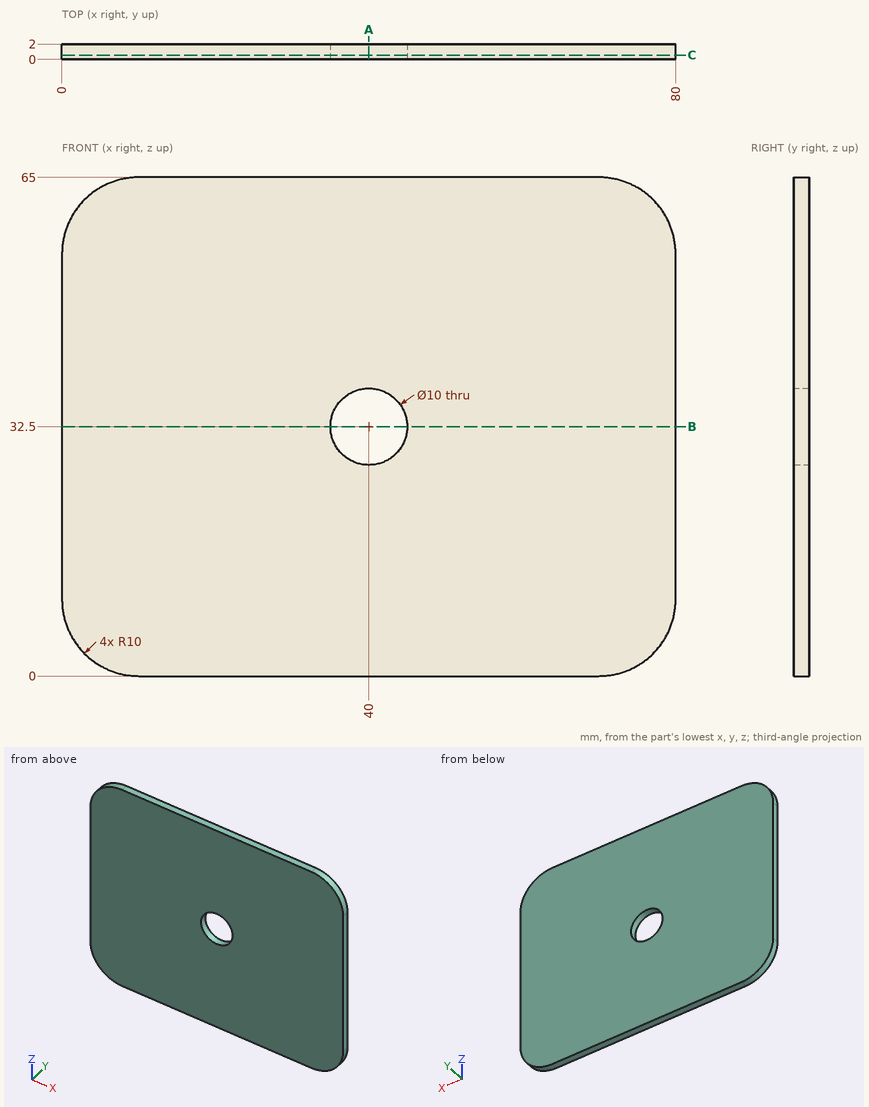
Design review of the part shown in the three views and the two pictorial views. Dimensions are in mm from the part's minimum x, y and z. Round coordinates to 2 decimals unless told otherwise and drop trailing zeros. Order: outer loops, then holes, each group sorted by start corner. A loop starts at its lowest first (then second) coordinate and runs counter-clockwise, first axis right, second up.
(1) For P1, Ø8, axis at x = 40, z = 32.5, coming from the -Y side, flat-tipped, find the tip position at first contact; note if it passes through.
Working result:
P1: passes through
(2) Take a section at A-A, the plane x = 40. State the section outline as (y, z) points, plus the area to 3 significant figures.
Working result:
outline: (0, 0) - (2, 0) - (2, 27.5) - (0, 27.5) - close; (0, 37.5) - (2, 37.5) - (2, 65) - (0, 65) - close
area: 110 mm2
(3) Wall thickness on L1, parallel to X at y = 1.3, z = 32.5; L2, parallel to Z at x = 37.5, y = 0.25; L3, parallel to Z at x = 6.5, y = 0.8: over which ranges is each line inside the solid? List them lowest first.
Working result:
L1: x = 0 to 35, 45 to 80
L2: z = 0 to 28.17, 36.83 to 65
L3: z = 0.63 to 64.37
(4) Take a section at B-B, the plane z = 32.5. State the section outline as (x, y) points, plus the area to 3 significant figures.
Working result:
outline: (0, 0) - (35, 0) - (35, 2) - (0, 2) - close; (45, 0) - (80, 0) - (80, 2) - (45, 2) - close
area: 140 mm2
(5) Take a section at C-C, the plane y = 0.55. State the section outline as (x, z) points.
Working result:
outline: (0, 10) arc R10 ccw to (10, 0) - (70, 0) arc R10 ccw to (80, 10) - (80, 55) arc R10 ccw to (70, 65) - (10, 65) arc R10 ccw to (0, 55) - close; hole circle Ø10 at (40, 32.5)
